Build history of the part. All positions in model axes, mm. A direction names the side the tool comes from. Round coordinates to 2 decimals unless told otherwise and drop trailing zeros. Write each loop counter-clockwise with the first axis right and the second up, starting at its lowest first coordinate (ties: lowest second). Pieces come first, ordered by that corner, then holes.
Item 1: Drop flat-ended pins along their axis: pin 1 Ø1.9 at (x, z) = (9.5, 0.5) entering from +Y; pin 2 Ø2.5 at (x, z) = (0, -1) entering from -Y; pin 3 Ø2 at (y, z) = (2, -0.5) entering from -X; pin 4 Ø1.5 at (x, z) = (13.5, 0) entering from -Y. Give the stop position or say it passes through.
Item 2: Band-saw the part on D-D, the plane y = -1.1. Write the cut outline in (x, z).
Item 3: Wall check: probe 1 along Z at (x, y) = (-11.5, 2); probe 2 along Y at (x, z) = (9, -0.5); probe 3 along Z at (x, y) = (16, 2.05). Give the ranges that are in metal, low to high.
Item 4: Band-saw the part on C-C, the plane z = 0. Count the separate pieces of the cut face and the enclosed holes in it, then the cut area to 3 significant figures.
Item 5: Band-saw the part on A-A, the plane x = 0. Write the cut outline in (y, z).
Item 6: 3-axis set-ups, long thin cutter, end or side, ignore diameter. For faces 1 (the cylindrical face through (-7.856, 1.486, -0.085)), 2 (the flat face through (-1, 1.4, -1)), 3 (the flat face through (3, -1.5, -1)), 4 (the cylindrical face through (2.44, 2.99, 0.54)), 5 (the flat face through (-4, 3, -0.6)): which of +Z, -Z, +X, -X, +Y, -Y reach the whole face in a straight line?
Item 7: Mould opens along X. For faces 6 (the cylindrical face through (16.55, 1.49, 0.35)), 7 (the flat face through (4, 3, -0.6)), 8 (the cylindrical face through (-18, 1, 0)) say: +X half, -X half, draft (parallel to the pull), parting line (faces both ways), or undercut.
Item 8: Band-saw the part on B-B, the plane x = 6. Write the cut outline in (y, z), then the cut area to 3 significant figures.
```python
from build123d import *
from OCP.BRepFilletAPI import BRepFilletAPI_MakeChamfer
from build123d.topology import SkipClean

# Parameters (mm, degrees)
SKETCH_1_R            = 0.65
SKETCH_1_R_2          = 1
EXTRUDE_1_DEPTH       = 2
EXTRUDE_START         = 1.5
SKETCH_2_R            = 3.75
SKETCH_2_R_2          = 1
EXTRUDE_2_DEPTH       = 1.5
SKETCH_3_R            = 3.75
SKETCH_3_R_2          = 1
EXTRUDE_3_DEPTH       = 1.5
EXTRUDE_4_DEPTH       = 1
SKETCH_5_R            = 2.5
CUT_EXTRUDE_1_DEPTH   = 2.5
CUT_EXTRUDE_START     = -1.5
SKETCH_6_R            = 2.5
CUT_EXTRUDE_2_DEPTH   = 1.5
MIRROR_2_COPY_1_DEPTH = 1
SKETCH_7_W            = 2.19635709
SKETCH_7_H            = 1.2
EXTRUDE_5_DEPTH       = 1.5
CHAMFER_1_SIZE        = 1.5
CHAMFER_1_SIZE_2      = 1
SKETCH_8_R            = 1
SKETCH_8_R_2          = 0.65
EXTRUDE_6_DEPTH       = 0.5
CUT_EXTRUDE_3_DEPTH   = 0.5
SKETCH_10_R           = 2.5
CUT_EXTRUDE_4_DEPTH   = 1.4
SKETCH_11_R           = 2.65
CUT_EXTRUDE_5_DEPTH   = 2.9


with BuildPart() as part:
    # 草图1 → 凸台-拉伸1 (new body)
    with BuildSketch(Plane(origin=(0, 0, 0), x_dir=(1, 0, 0), z_dir=(0, 1, 0))):
        with BuildLine():
            Line((0.41015625, 3.727502093), (16.21875, 1.988001116))
            ThreePointArc((16.21875, 1.988001116), (18, 0), (16.21875, -1.988001116))
            Line((16.21875, -1.988001116), (0.41015625, -3.727502093))
            ThreePointArc((0.41015625, -3.727502093), (-3.75, 0), (0.41015625, 3.727502093))
        make_face()
        with Locations(Location((16, 0, 0), (0, 0, 270))):
            Circle(SKETCH_1_R, mode=Mode.SUBTRACT)
        with Locations(Location((6, 0, 0), (0, 0, 270))):
            Circle(SKETCH_1_R, mode=Mode.SUBTRACT)
        with Locations(Location((8.5, 0, 0), (0, 0, 270))):
            Circle(SKETCH_1_R, mode=Mode.SUBTRACT)
        with Locations(Location((11, 0, 0), (0, 0, 270))):
            Circle(SKETCH_1_R, mode=Mode.SUBTRACT)
        with Locations(Location((13.5, 0, 0), (0, 0, 270))):
            Circle(SKETCH_1_R, mode=Mode.SUBTRACT)
        with Locations(Location((0, 0, 0), (0, 0, 270))):
            Circle(SKETCH_1_R_2, mode=Mode.SUBTRACT)
    extrude_1 = extrude(amount=EXTRUDE_1_DEPTH)

    # 草图2 → 凸台-拉伸2 (add)
    with SkipClean():  # the faces are left unmerged after this step: merging them gives an invalid solid
        with BuildSketch(Plane.XZ.offset(EXTRUDE_START)):
            with Locations(Location((0, 0, 0), (0, 0, 270))):
                Circle(SKETCH_2_R)
            with Locations(Location((0, 0, 0), (0, 0, 270))):
                Circle(SKETCH_2_R_2, mode=Mode.SUBTRACT)
        extrude(amount=-EXTRUDE_2_DEPTH)

    # 草图3 → 凸台-拉伸3 (add)
    with SkipClean():  # the faces are left unmerged after this step: merging them gives an invalid solid
        with BuildSketch(Plane(origin=(0, 2, 0), x_dir=(1, 0, 0), z_dir=(0, 1, 0))):
            with Locations(Location((0, 0, 0), (0, 0, 90))):
                Circle(SKETCH_3_R)
            with Locations(Location((0, 0, 0), (0, 0, 90))):
                Circle(SKETCH_3_R_2, mode=Mode.SUBTRACT)
        extrude(amount=EXTRUDE_3_DEPTH)

    # 草图4 → 凸台-拉伸4 (add)
    with SkipClean():  # the faces are left unmerged after this step: merging them gives an invalid solid
        with BuildSketch(Plane(origin=(0.41015625, 0, 3.727502093), x_dir=(0.9940005580355578, 0, -0.10937499999999994), z_dir=(0.10937499999999994, 0, 0.9940005580355578))):
            Polygon((0, 2), (0, 3.5), (3.75, 3.5), (5.25, 2), align=None)
        extrude_4 = extrude(amount=-EXTRUDE_4_DEPTH)

    # 镜向1: 凸台-拉伸4 across plane
    with SkipClean():  # the faces are left unmerged after this step: merging them gives an invalid solid
        add(extrude_4.mirror(Plane.XY))

    # 草图5 → 切除-拉伸1 (cut)
    with SkipClean():  # the faces are left unmerged after this step: merging them gives an invalid solid
        with BuildSketch(Plane.XZ.offset(1.5)):
            with Locations(Location((0, 0, 0), (0, 0, 270))):
                Circle(SKETCH_5_R)
        extrude(amount=-CUT_EXTRUDE_1_DEPTH, mode=Mode.SUBTRACT)

    # 草图6 → 切除-拉伸2 (cut)
    with SkipClean():  # the faces are left unmerged after this step: merging them gives an invalid solid
        with BuildSketch(Plane(origin=(0, 3.5, 0), x_dir=(1, 0, 0), z_dir=(0, 1, 0)).offset(CUT_EXTRUDE_START)):
            with Locations(Location((0, 0, 0), (0, 0, 90))):
                Circle(SKETCH_6_R)
        extrude(amount=CUT_EXTRUDE_2_DEPTH, mode=Mode.SUBTRACT)

    # 镜向2: 凸台-拉伸1, 凸台-拉伸4 across plane
    with SkipClean():  # the faces are left unmerged after this step: merging them gives an invalid solid
        add(extrude_1.mirror(Plane(origin=(0, 0, 0), x_dir=(0, 0, 1), z_dir=(1, 0, 0))))
        add(extrude_4.mirror(Plane(origin=(0, 0, 0), x_dir=(0, 0, 1), z_dir=(1, 0, 0))))

    # 镜向2 copy 1 sketch → 镜向2 copy 1 (add)
    with SkipClean():  # the faces are left unmerged after this step: merging them gives an invalid solid
        with BuildSketch(Plane(origin=(-0.41015625, 0, -3.727502093), x_dir=(-0.9940005580355578, 0, 0.10937499999999994), z_dir=(-0.10937499999999994, 0, -0.9940005580355578))):
            Polygon((0, 2), (0, 3.5), (3.75, 3.5), (5.25, 2), align=None)
        extrude(amount=-MIRROR_2_COPY_1_DEPTH)

    # 草图7 → 凸台-拉伸5 (add)
    with SkipClean():  # the faces are left unmerged after this step: merging them gives an invalid solid
        with BuildSketch(Plane(origin=(0, 3.5, 0), x_dir=(1, 0, 0), z_dir=(0, 1, 0))):
            with Locations((3.75, 0)):
                Rectangle(SKETCH_7_W, SKETCH_7_H)
            with Locations((-3.75, 0)):
                Rectangle(SKETCH_7_W, SKETCH_7_H)
        extrude(amount=-EXTRUDE_5_DEPTH)

    # 倒角1
    chamfer_1_edges_1 = [part.edges().sort_by_distance(p)[0] for p in [
        (4.848178545, 3.5, 0),
    ]]
    chamfer_1_side_1 = [part.faces().sort_by_distance(p)[0] for p in [
        (4.848178545, 3.48, 0),
    ]]
    chamfer_1_edges_2 = [part.edges().sort_by_distance(p)[0] for p in [
        (-4.848178545, 3.5, 0),
    ]]
    chamfer_1_side_2 = [part.faces().sort_by_distance(p)[0] for p in [
        (-4.848178545, 3.48, 0),
    ]]
    chamfer_1 = BRepFilletAPI_MakeChamfer(part.part.solid().wrapped)
    for e in chamfer_1_edges_1:
        chamfer_1.Add(CHAMFER_1_SIZE - 0.0001, CHAMFER_1_SIZE_2 - 0.0001, e.wrapped, chamfer_1_side_1[0].wrapped)
    for e in chamfer_1_edges_2:
        chamfer_1.Add(CHAMFER_1_SIZE - 0.0001, CHAMFER_1_SIZE_2 - 0.0001, e.wrapped, chamfer_1_side_2[0].wrapped)
    add(Compound.cast(chamfer_1.Shape()), mode=Mode.REPLACE)  # a hair under: the kernel refuses the full size

    # 草图8 → 凸台-拉伸6 (add)
    with BuildSketch(Plane(origin=(0, 2, 0), x_dir=(1, 0, 0), z_dir=(0, 1, 0))):
        with BuildLine():
            Line((-5.62865918, -3.153283343), (-16.21875, -1.988001116))
            ThreePointArc((-16.21875, -1.988001116), (-18, 0), (-16.21875, 1.988001116))
            Line((-16.21875, 1.988001116), (-5.62865918, 3.153283343))
            Line((-5.62865918, 3.153283343), (-4.137658343, 3.317345843))
            Line((-4.137658343, 3.317345843), (-0.41015625, 3.727502093))
            ThreePointArc((-0.41015625, 3.727502093), (0, 3.75), (0.41015625, 3.727502093))
            Line((0.41015625, 3.727502093), (4.137658343, 3.317345843))
            Line((4.137658343, 3.317345843), (5.62865918, 3.153283343))
            Line((5.62865918, 3.153283343), (16.21875, 1.988001116))
            ThreePointArc((16.21875, 1.988001116), (18, 0), (16.21875, -1.988001116))
            Line((16.21875, -1.988001116), (5.62865918, -3.153283343))
            Line((5.62865918, -3.153283343), (4.137658343, -3.317345843))
            Line((4.137658343, -3.317345843), (0.41015625, -3.727502093))
            ThreePointArc((0.41015625, -3.727502093), (0, -3.75), (-0.41015625, -3.727502093))
            Line((-0.41015625, -3.727502093), (-4.137658343, -3.317345843))
            Line((-4.137658343, -3.317345843), (-5.62865918, -3.153283343))
        make_face()
        with Locations(Location((0, 0, 0), (0, 0, 270))):
            Circle(SKETCH_8_R, mode=Mode.SUBTRACT)
        with Locations(Location((16, 0, 0), (0, 0, 270))):
            Circle(SKETCH_8_R_2, mode=Mode.SUBTRACT)
        with Locations(Location((13.5, 0, 0), (0, 0, 270))):
            Circle(SKETCH_8_R_2, mode=Mode.SUBTRACT)
        with Locations(Location((11, 0, 0), (0, 0, 270))):
            Circle(SKETCH_8_R_2, mode=Mode.SUBTRACT)
        with Locations(Location((8.5, 0, 0), (0, 0, 270))):
            Circle(SKETCH_8_R_2, mode=Mode.SUBTRACT)
        with Locations(Location((6, 0, 0), (0, 0, 270))):
            Circle(SKETCH_8_R_2, mode=Mode.SUBTRACT)
        with Locations(Location((-6, 0, 0), (0, 0, 270))):
            Circle(SKETCH_8_R_2, mode=Mode.SUBTRACT)
        with Locations(Location((-8.5, 0, 0), (0, 0, 270))):
            Circle(SKETCH_8_R_2, mode=Mode.SUBTRACT)
        with Locations(Location((-11, 0, 0), (0, 0, 270))):
            Circle(SKETCH_8_R_2, mode=Mode.SUBTRACT)
        with Locations(Location((-13.5, 0, 0), (0, 0, 270))):
            Circle(SKETCH_8_R_2, mode=Mode.SUBTRACT)
        with Locations(Location((-16, 0, 0), (0, 0, 270))):
            Circle(SKETCH_8_R_2, mode=Mode.SUBTRACT)
    extrude(amount=EXTRUDE_6_DEPTH)

    # 草图9 → 切除-拉伸3 (cut)
    with BuildSketch(Plane.XZ):
        with BuildLine():
            Line((0.41015625, -3.727502093), (16.21875, -1.988001116))
            ThreePointArc((16.21875, -1.988001116), (18, 0), (16.21875, 1.988001116))
            Line((16.21875, 1.988001116), (0.41015625, 3.727502093))
            ThreePointArc((0.41015625, 3.727502093), (3.75, 0), (0.41015625, -3.727502093))
        make_face()
        with BuildLine():
            Line((-16.21875, -1.988001116), (-0.41015625, -3.727502093))
            ThreePointArc((-0.41015625, -3.727502093), (-3.75, 0), (-0.41015625, 3.727502093))
            Line((-0.41015625, 3.727502093), (-16.21875, 1.988001116))
            ThreePointArc((-16.21875, 1.988001116), (-18, 0), (-16.21875, -1.988001116))
        make_face()
    extrude(amount=-CUT_EXTRUDE_3_DEPTH, mode=Mode.SUBTRACT)

    # 草图10 → 切除-拉伸4 (cut)
    with BuildSketch(Plane.XZ):
        with Locations(Location((0, 0, 0), (0, 0, 270))):
            Circle(SKETCH_10_R)
    extrude(amount=-CUT_EXTRUDE_4_DEPTH, mode=Mode.SUBTRACT)

    # 草图11 → 切除-拉伸5 (cut)
    with BuildSketch(Plane.XZ.offset(1.5)):
        with Locations(Location((0, 0, 0), (0, 0, 270))):
            Circle(SKETCH_11_R)
    extrude(amount=-CUT_EXTRUDE_5_DEPTH, mode=Mode.SUBTRACT)


solid = part.part
```
Results:
1. pin 1: stops at y = 2.5
1. pin 2: stops at y = 1.4
1. pin 3: stops at x = -18
1. pin 4: stops at y = 0.5
2. outline: circle Ø7.5 at (0, 0); hole circle Ø5.3 at (0, 0)
3. probe 1: z = -2.51 to -0.42, 0.42 to 2.51
3. probe 2: y = 0.5 to 2.5
3. probe 3: z = -2.01 to -0.65, 0.65 to 2.01
4. separate pieces: 12
4. enclosed holes: 0
4. area: 46.8 mm2
5. outline: (-1.5, -3.75) - (3.5, -3.75) - (3.5, -2.5) - (2.5, -2.5) - (2.5, -1) - (1.4, -1) - (1.4, -2.65) - (-1.5, -2.65) - close; (-1.5, 2.65) - (1.4, 2.65) - (1.4, 1) - (2.5, 1) - (2.5, 2.5) - (3.5, 2.5) - (3.5, 3.75) - (-1.5, 3.75) - close
6. face 1: +Y, -Y
6. face 2: -Y
6. face 3: +Z, -Z, +X, -X, -Y
6. face 4: +Y
6. face 5: -X, +Y
7. face 6: undercut
7. face 7: draft
7. face 8: -X half
8. outline: (0.5, -3.11) - (2.5, -3.11) - (2.5, -0.65) - (0.5, -0.65) - close; (0.5, 0.65) - (2.5, 0.65) - (2.5, 3.11) - (0.5, 3.11) - close
8. area: 9.85 mm2
